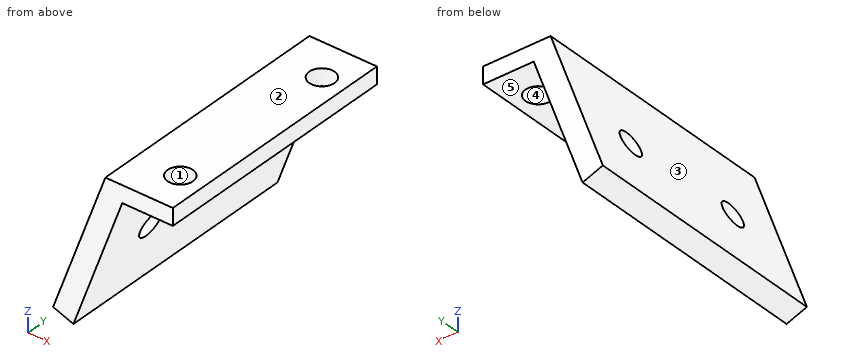
```python
from build123d import *

# Parameters (mm, degrees)
BOSS_EXTRUDE1_DEPTH = 30
SKETCH2_R           = 1.5
CUT_EXTRUDE1_DEPTH  = 30
SKETCH3_R           = 1.5
CUT_EXTRUDE2_DEPTH  = 30


with BuildPart() as part:
    # Sketch1 → Boss-Extrude1 (new body)
    with BuildSketch(Plane(origin=(0, 0, 0), x_dir=(1, 0, 0), z_dir=(0, 1, 0))):
        Polygon((-4.53610988, -6.260301285), (3.46389012, -6.260301285), (3.46389012, -4.260301285), (-2.53610988, -4.260301285), (-8.328469686, 11.654076488), (-10.737301739, 10.777333321), align=None)
    extrude(amount=BOSS_EXTRUDE1_DEPTH)

    # Sketch2 → Cut-Extrude1 (cut)
    with BuildSketch(Plane(origin=(0, 0, 4.260301285), x_dir=(-1, 0, 0), z_dir=(0, 0, -1))):
        with Locations((-0.63889012, 25.414)):
            Circle(SKETCH2_R)
        with Locations((-0.64389012, 4.59)):
            Circle(SKETCH2_R)
    extrude(amount=-CUT_EXTRUDE1_DEPTH, mode=Mode.SUBTRACT)

    # Sketch3 → Cut-Extrude2 (cut)
    with BuildSketch(Plane(origin=(-2.53610988, 0, 0), x_dir=(0, 0, -1), z_dir=(1, 0, 0))):
        with Locations(Location((3.239698715, 22.5, 0), (0, 0, 180))):
            Circle(SKETCH3_R)
        with Locations(Location((3.239698715, 7.5, 0), (0, 0, 180))):
            Circle(SKETCH3_R)
    extrude(amount=-CUT_EXTRUDE2_DEPTH, mode=Mode.SUBTRACT)


solid = part.part
```
The listing builds one solid part. Answer for the finished solid, in the listing's coordinates (mm). Face numbers are marked on the shaded views. A direction names the side the tool comes from. Give positions to 0.01 mm unless a question says otherwise; leave off trailing zeros. Order: outer loops, then holes, each group sorted by start corner. A loop starts at its lowest first (then second) coordinate and runs counter-clockwise, first axis right, second up. Notation, with made-up numbers: (45, 43.25) -> (49, 43.25) arc R24 cw to (49, 63.25) -> close; hole circle Ø8 at (17, 34.25). An arc over 180 degrees is marked (long way). Answer as CSV lines item,"result". Start each with the question number.
Q1. A cutting plane is placed at D-D (z = 5.25). Determine the outline of the cut face in (x, y), then the cut area to 3 significant figures.
Q2. A cutting plane is placed at A-A (y = 4.59). Determine the outline of the cut face in (x, z).
Q3. Which of the six approach directions +Z, -Z, +X, -X, +Y, -Y give full straight-line access (tool end or side, diameter ignored) to the marked faces 4 and 5?
Q4. Given pin 1 (1.8 mm diameter, centred on y = 22.5, z = -3.24, fed in from -X); pin 2 (10 mm diameter, centred on y = 9, z = 0, fed in from -X); pin 3 (1.5 mm diameter, centred on y = 26.5, z = -8.5, fed in from -X); pin 4 (4 mm diameter, centred on x = 0.64, y = 25.41, fed in from -Z), each flat-ended and moving along its own axis, determine where each tip first touches the part or whether it passes through.
Q5. Determine the mould class of the marked faces 1, 2 and 3 for opening direction X: pulls with the +X half, pulls with the -X half, needs draft (parallel to the pull), parting line crosses it, or undercut.
Q6. Find the intervals of material crossed by L1, parallel to Z at x = -0.5, y = 5.75; L2, parallel to Y at x = -6.75, z = -2; L3, parallel to X at y = 1.5, z = -1.5, in increasing order.
Q7. A cutting plane is placed at C-C (y = 10.25). Determine the outline of the cut face in (x, z).
Q8. A cutting plane is placed at B-B (z = -2.75). Determine the outline of the cut face in (x, y).
Results found:
1,outline,"(-4.9, 0) -> (3.46, 0) -> (3.46, 30) -> (-4.9, 30) -> close; hole circle Ø3 at (0.64, 4.59); hole circle Ø3 at (0.64, 25.41)"
1,area,"237 mm2"
2,outline,"(-10.74, -10.78) -> (-8.33, -11.65) -> (-2.54, 4.26) -> (-0.86, 4.26) -> (-0.86, 6.26) -> (-4.54, 6.26) -> close; (2.14, 4.26) -> (3.46, 4.26) -> (3.46, 6.26) -> (2.14, 6.26) -> close"
3,face 4,"+Z, -Z"
3,face 5,"-Z, +X, +Y, -Y"
4,pin 1,"through"
4,pin 2,"x = -8.63"
4,pin 3,"x = -10.18"
4,pin 4,"z = 4.26"
5,face 1,"undercut"
5,face 2,"needs draft"
5,face 3,"pulls with the -X half"
6,L1,"4.26 to 6.26"
6,L2,"0 to 6.66, 8.34 to 21.66, 23.34 to 30"
6,L3,"-7.36 to -4.63"
7,outline,"(-10.74, -10.78) -> (-8.33, -11.65) -> (-2.54, 4.26) -> (3.46, 4.26) -> (3.46, 6.26) -> (-4.54, 6.26) -> close"
8,outline,"(-7.82, 0) -> (-5.09, 0) -> (-5.09, 6.08) -> (-7.82, 6.08) -> close; (-7.82, 8.92) -> (-5.09, 8.92) -> (-5.09, 21.08) -> (-7.82, 21.08) -> close; (-7.82, 23.92) -> (-5.09, 23.92) -> (-5.09, 30) -> (-7.82, 30) -> close"
